Design review of the part built by this model. Coordinates are the model's own, in mm. Face numbers are marked on the shaded views. A direction names the side the tool comes from. Give positions to 0.01 mm unless a question says otherwise; leave off trailing zeros. Order: outer loops, then holes, each group sorted by start corner. A loop starts at its lowest first (then second) coordinate and runs counter-clockwise, first axis right, second up.
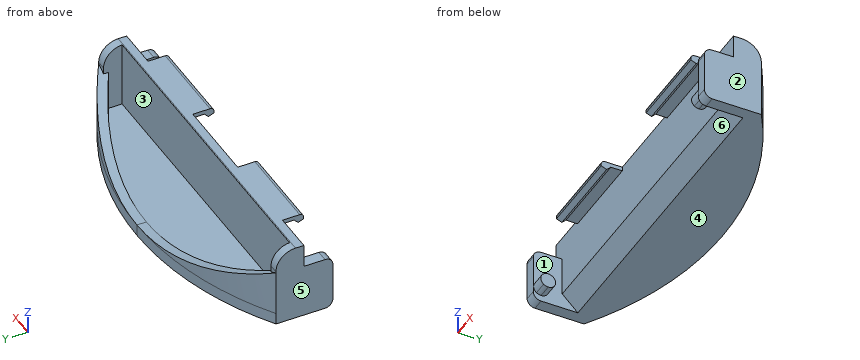
```python
from build123d import *

# Parameters (mm, degrees)
F1_DEPTH  = 3
F3_DEPTH  = 17
F5_DEPTH  = 17.6
F6_W      = 3
F6_H      = 14
F7_DEPTH  = 7.4
F8_R      = 2
F6_W_2    = 22
F6_H_2    = 2.1
F9_DEPTH  = 5.4
F10_R     = 1
F12_SIZE  = 4
F14_DEPTH = 3.5
F18_DEPTH = 66
F20_DEPTH = 4.7397795647
F21_F1_R  = 4.9999


# Not quite as in the source:
# - a fillet or chamfer is up to 0.001 mm smaller than in the source, because OpenCascade refuses the exact size


with BuildPart() as f1:
    # F0 (on Top) → F1 (new body)
    with BuildSketch(Plane.XY):
        with BuildLine():
            Line((43.5, -20), (43.5, 0))
            ThreePointArc((43.5, 0), (20.8194176131, -3.2823932686), (0, -12.8602204353))
            Line((0, -12.8602204353), (0, -20))
            Line((0, -20), (43.5, -20))
        make_face()
        with BuildLine():
            ThreePointArc((87, -12.8602204353), (66.1805823869, -3.2823932686), (43.5, 0))
            Line((43.5, 0), (43.5, -20))
            Line((43.5, -20), (87, -20))
            Line((87, -20), (87, -12.8602204353))
        make_face()
    extrude(amount=F1_DEPTH)

    # F2 (on face) → F3 (join)
    with BuildSketch(Plane.XY.offset(3)):
        with BuildLine():
            ThreePointArc((87, -12.8602204353), (43.5, 0), (0, -12.8602204353))
            Line((0, -12.8602204353), (0, -20))
            Line((0, -20), (87, -20))
            Line((87, -20), (87, -12.8602204353))
        make_face()
        with BuildLine():
            Line((84.6, -17.6), (2.4, -17.6))
            Line((2.4, -17.6), (2.4, -14.1778912523))
            ThreePointArc((2.4, -14.1778912523), (43.5, -2.4), (84.6, -14.1778912523))
            Line((84.6, -14.1778912523), (84.6, -17.6))
        make_face(mode=Mode.SUBTRACT)
    extrude(amount=F3_DEPTH)

    # F4 (on Front) → F5 (cut, through all)
    with BuildSketch(Plane.XZ):
        with BuildLine():
            ThreePointArc((130.5, 90), (-18.0182899632, 151.5182899632), (43.5, 3))
            ThreePointArc((43.5, 3), (105.0182899632, 28.4817100368), (130.5, 90))
        make_face()
    extrude(amount=F5_DEPTH, mode=Mode.SUBTRACT)

    # F6 (on face) → F7 (join)
    with BuildSketch(Plane.XZ.offset(20)):
        with Locations((1.5, 7)):
            Rectangle(F6_W, F6_H)
        with Locations((85.5, 7)):
            Rectangle(F6_W, F6_H)
    extrude(amount=F7_DEPTH)

    # F8
    f8_edges = [f1.edges().sort_by_distance(p)[0] for p in [
        (1.5, -27.4, 0),
        (1.5, -27.4, 14),
        (85.5, -27.4, 14),
        (85.5, -27.4, 0),
    ]]
    fillet(f8_edges, radius=F8_R)

    # F6 (on face) → F9 (join)
    with BuildSketch(Plane.XZ.offset(20)):
        with Locations((21.5, 18.95)):
            Rectangle(F6_W_2, F6_H_2)
        with Locations((65.5, 18.95)):
            Rectangle(F6_W_2, F6_H_2)
    extrude(amount=F9_DEPTH)

    # F10
    f10_edges = [f1.edges().sort_by_distance(p)[0] for p in [
        (21.5, -25.4, 20),
        (65.5, -25.4, 20),
    ]]
    fillet(f10_edges, radius=F10_R)

    # F12
    f12_edges = [f1.edges().sort_by_distance(p)[0] for p in [
        (43.5, -20, 0),
    ]]
    chamfer(f12_edges, length=F12_SIZE)

    # F13 (on face) → F14 (join)
    with BuildSketch(Plane.YZ.offset(3)):
        with BuildLine():
            Line((-25.4, 2), (-26.566190379, 2))
            ThreePointArc((-26.566190379, 2), (-26.0164414003, 1.7027799244), (-25.4, 1.6))
            Line((-25.4, 1.6), (-25.4, 2))
        make_face()
        with BuildLine():
            ThreePointArc((-23.5, 3.5), (-26.2349366084, 5.2067163971), (-26.566190379, 2))
            Line((-26.566190379, 2), (-25.4, 2))
            Line((-25.4, 2), (-25.4, 1.6))
            ThreePointArc((-25.4, 1.6), (-24.0564971157, 2.1564971157), (-23.5, 3.5))
        make_face()
    extrude(amount=F14_DEPTH)

    # F17: F1 across plane


with BuildPart() as f1_1:
    add(f1.part)
    add(f1.part.mirror(Plane.YZ.offset(43.5)))

    # F11 (on face) → F18 (cut, through all)
    with BuildSketch(Plane(origin=(10.5, 0, 0), x_dir=(0, -1, 0), z_dir=(-1, 0, 0))):
        Polygon((22.95, 18.95), (20, 18.95), (20, 17.9), (24, 17.9), align=None)
        Polygon((25.4, 17.9), (25.4, 18.45), (24, 17.9), align=None)
    extrude(amount=-F18_DEPTH, mode=Mode.SUBTRACT)

    # F19 (on face) → F20 (join, through all)
    with BuildSketch(Plane(origin=(0, -17.6, 0), x_dir=(-1, 0, 0), z_dir=(0, 1, 0))):
        with BuildLine():
            Line((-84.6, 13.3202112679), (-84.6, 20))
            Line((-84.6, 20), (-87, 20))
            Line((-87, 20), (-87, 14.6557898708))
            ThreePointArc((-87, 14.6557898708), (-85.8052708602, 13.9785289708), (-84.6, 13.3202112679))
        make_face()
        with BuildLine():
            Line((-2.4, 20), (-2.4, 13.3202112679))
            ThreePointArc((-2.4, 13.3202112679), (-1.1947291398, 13.9785289708), (0, 14.6557898708))
            Line((0, 14.6557898708), (0, 20))
            Line((0, 20), (-2.4, 20))
        make_face()
    extrude(amount=F20_DEPTH)

    # F21: fillet of radius 5 on 2 edges, made by hand

    # F21_f1 (radius 5 in the source; OpenCascade refuses exactly that, so slightly less here)
    f21_f1_edges = [f1_1.edges().sort_by_distance(p)[0] for p in [
        (85.8, -12.8602204353, 20),
    ]]
    fillet(f21_f1_edges, radius=F21_F1_R)


solid = f1_1.part
```
1. For line 1 along X through (y, z) = (-22.5, 8.25); line 2 along X through (y, z) = (-17.25, 16.75); line 3 along Z through (x, y) = (7.5, -12.5), list the stretches that pass through material, from the lowest coordinate up.
Recorded:
line 1: x = 0 to 3, 84 to 87
line 2: x = 0 to 2.4, 84.6 to 87
line 3: z = 0 to 3
2. Take a section at C-C (x = 17.5). State the section outline as (y, z) points.
Recorded:
outline: (-25.4, 18.45) - (-24, 17.9) - (-22.95, 18.95) - (-20, 18.95) - (-20, 4) - (-16, 0) - (-4.34, 0) - (-4.34, 6.98) - (-6.89, 6.98) - (-6.89, 3) - (-17.6, 3) - (-17.6, 19.99) arc R5 ccw to (-17.86, 20) - (-24.4, 20) arc R1 ccw to (-25.4, 19) - close
3. For pin 1 (1.3 mm diameter, centred on x = 85.5, z = 14, fed in from +Y); pin 2 (3 mm diameter, centred on x = 67.5, y = -21, fed in from -Z); pin 3 (1.1 mm diameter, centred on y = -21.5, z = 19, fed in from -X), all flat-tipped, find the tip position at first contact; note any pin that passes through.
Recorded:
pin 1: stops at y = -11.62
pin 2: stops at z = 3.5
pin 3: stops at x = 10.5
4. Take a section at D-D (y = -15). State the section outline as (x, z) points, then the cut area to 3 significant figures.
Recorded:
outline: (0, 0) - (87, 0) - (87, 19.1) - (84.6, 19.1) - (84.6, 3) - (2.4, 3) - (2.4, 19.1) - (0, 19.1) - close
area: 338 mm2
5. Draft analysis for pull direction X (two halves, no side actions). For the marked faces 4, 5 and 6, state which applies: pulls with the +X half, pulls with the -X half, needs draft (parallel to the pull), parting line crosses it, or undercut.
Recorded:
face 4: needs draft
face 5: pulls with the -X half
face 6: undercut
6. Take a section at A-A (y = -21.25). State the section outline as (x, z) points, then the cut area to 3 significant figures.
Recorded:
outline: (0, 0) - (3, 0) - (3, 14) - (0, 14) - close; (10.5, 18.95) - (32.5, 18.95) - (32.5, 20) - (10.5, 20) - close; (54.5, 18.95) - (76.5, 18.95) - (76.5, 20) - (54.5, 20) - close; (84, 0) - (87, 0) - (87, 14) - (84, 14) - close
area: 130 mm2
7. Take a section at B-B (z = 16.5). State the section outline as (x, y) points.
Recorded:
outline: (0, -20) - (87, -20) - (87, -13.09) - (84.6, -13.09) - (84.6, -17.6) - (2.4, -17.6) - (2.4, -13.09) - (0, -13.09) - close
8. Machinability: for the marked faces 1, 2 and 3, which of the approach directions +Z, -Z, +X, -X, +Y, -Y give a long, thin tool a straight path to every point of the face, cutting with its end or side? Answer none if there is none.
Recorded:
face 1: none
face 2: +Z, -Z, +X, +Y, -Y
face 3: +Z
